Geometry: final body of the model. Coordinates: model frame, mm. Face numbers are marked on the shaded views. Give positions to 0.01 mm unless a question says otherwise; leave off trailing zeros. Write each loop counter-clockwise with the first axis right and the second up, starting at its lowest first coordinate (ties: lowest second). Pieces come first, ordered by that corner, then holes. Notation, with made-up numbers: (13, 19.25) -> (35, 19.25) arc R8 cw to (35, 25.25) -> close; hole circle Ø6 at (-12, 63.5). An arc over 180 degrees is marked (long way). Answer as a JSON object with one key per item and string values.
from build123d import *

# Parameters (mm, degrees)
PAD011_DEPTH    = 30
PAD012_DEPTH    = 0.8
PAD013_DEPTH    = 1.7
PAD014_DEPTH    = 3
CHAMFER002_SIZE = 1.5


with BuildPart() as part:
    # Sketch014 → Pad011 (new body, symmetric)
    with BuildSketch(Plane.YZ):
        with BuildLine():
            ThreePointArc((-13.5, 21.519943), (-21.311021, 27.174165), (-29.878928, 22.75))
            Line((-31.3, 22.75), (-29.878928, 22.75))
            ThreePointArc((-31.3, 24.25), (-32.05, 23.5), (-31.3, 22.75))
            Line((-31.3, 26.5), (-31.3, 24.25))
            Line((-33, 26.5), (-31.3, 26.5))
            Line((-33, 26.5), (-33, 29))
            Line((9, 29), (-33, 29))
            Line((9, 26.5), (9, 29))
            Line((9, 26.5), (6.8, 26.5))
            Line((6.8, 26.5), (6.8, 24.25))
            ThreePointArc((6.8, 22.75), (7.55, 23.5), (6.8, 24.25))
            Line((5.878928, 22.75), (6.8, 22.75))
            ThreePointArc((5.878928, 22.75), (-2.688979, 27.174165), (-10.5, 21.519943))
            Line((-13.5, 21.519943), (-10.5, 21.519943))
        make_face()
    extrude(amount=PAD011_DEPTH, both=True)

    # Sketch015 (on Face9 of Pad011) → Pad012 (join)
    with BuildSketch(Plane(origin=(0, 0, 29), x_dir=(0, -1, 0), z_dir=(0, 0, 1))):
        with BuildLine():
            ThreePointArc((-6.999999, 37.5), (-8.414213, 36.914214), (-9, 35.5))
            Line((-9, 30), (-9, 35.5))
            Line((33, 30), (-9, 30))
            Line((33, 35.5), (33, 30))
            ThreePointArc((33, 35.5), (32.414214, 36.914214), (31, 37.5))
            Line((-6.999999, 37.5), (31, 37.5))
        make_face()
        with BuildLine():
            Line((-9, -30), (33, -30))
            Line((33, -30), (33, -36))
            ThreePointArc((31, -38), (32.414214, -37.414214), (33, -36))
            Line((-7, -38), (31, -38))
            ThreePointArc((-9, -36.000001), (-8.414213, -37.414214), (-7, -38))
            Line((-9, -30), (-9, -36.000001))
        make_face()
    extrude(amount=-PAD012_DEPTH)

    # Sketch016 (on Face15 of Pad012) → Pad013 (join)
    with BuildSketch(Plane.YX.offset(-28.2)):
        with BuildLine():
            Line((-31.3, 30), (-33, 30))
            Line((-33, 30), (-33, 35.5))
            ThreePointArc((-31, 37.5), (-32.414214, 36.914214), (-33, 35.5))
            Line((6.999999, 37.5), (-31, 37.5))
            ThreePointArc((9, 35.5), (8.414213, 36.914214), (6.999999, 37.5))
            Line((9, 30), (9, 35.5))
            Line((9, 30), (6.8, 30))
            Line((6.8, 30), (6.8, 35))
            ThreePointArc((6.8, 35), (6.507107, 35.707107), (5.8, 36))
            Line((5.8, 36), (-30.3, 36))
            ThreePointArc((-30.3, 36), (-31.007107, 35.707107), (-31.3, 35))
            Line((-31.3, 30), (-31.3, 35))
        make_face()
        with BuildLine():
            ThreePointArc((7, -38), (8.414213, -37.414214), (9, -36.000001))
            Line((9, -30), (9, -36.000001))
            Line((6.8, -30), (9, -30))
            Line((6.8, -30), (6.8, -35.5))
            ThreePointArc((5.8, -36.5), (6.507107, -36.207107), (6.8, -35.5))
            Line((-30.3, -36.5), (5.8, -36.5))
            ThreePointArc((-31.3, -35.5), (-31.007107, -36.207107), (-30.3, -36.5))
            Line((-31.3, -30), (-31.3, -35.5))
            Line((-33, -30), (-31.3, -30))
            Line((-33, -36), (-33, -30))
            ThreePointArc((-33, -36), (-32.414214, -37.414214), (-31, -38))
            Line((-31, -38), (7, -38))
        make_face()
    extrude(amount=PAD013_DEPTH)

    # Sketch018 (on Face20 of Pad013) → Pad014 (join)
    with BuildSketch(Plane.YX.offset(-28.2)):
        with BuildLine():
            Line((-31.3, 35), (6.8, 35))
            ThreePointArc((6.8, 35), (6.507107, 35.707107), (5.8, 36))
            Line((5.8, 36), (-30.3, 36))
            ThreePointArc((-30.3, 36), (-31.007107, 35.707107), (-31.3, 35))
        make_face()
        with BuildLine():
            ThreePointArc((5.8, -36.5), (6.507107, -36.207107), (6.8, -35.5))
            Line((-31.3, -35.5), (6.8, -35.5))
            ThreePointArc((-31.3, -35.5), (-31.007107, -36.207107), (-30.3, -36.5))
            Line((5.8, -36.5), (-30.3, -36.5))
        make_face()
    extrude(amount=PAD014_DEPTH)

    # Chamfer002
    chamfer002_edges = [part.edges().sort_by_distance(p)[0] for p in [
        (35, -12.25, 28.2),
        (-35.5, -12.25, 28.2),
    ]]
    chamfer(chamfer002_edges, length=CHAMFER002_SIZE)


solid = part.part
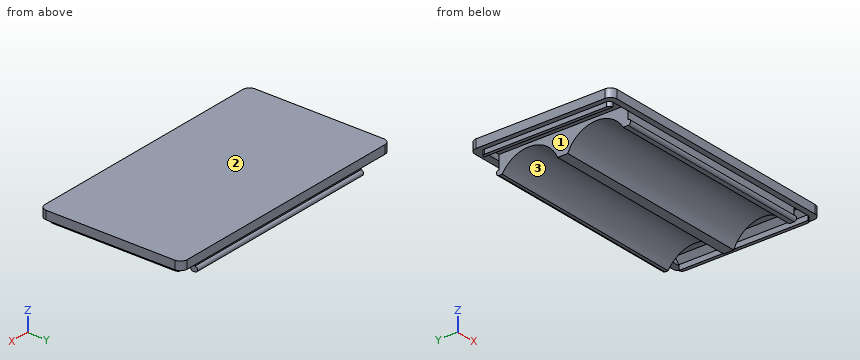
Q1. Material intervals for L1, parallel to X at y = -9, z = 25.5; L2, parallel to X at y = -23.5, z = 25.5; L3, parallel to Y at x = 13, z = 24.5, sorted ascending. Write a range as from..to.
Values:
{"L1": "-36.5..-35.5, -30..30, 35..36", "L2": "-36.5..-35.5, 35..36", "L3": "-31.3..-28.51, -15.49..-8.51, 4.51..6.8"}
Q2. First-contact query: P1, Ø4, axis at x = 19, z = 24, coming from the -Y side; P2, Ø0.7, axis at x = 5, z = 26, coming from the -Y side; P3, Ø1.8, axis at x = -13.5, z = 25, coming from the +Y side. Flat tips, straight axial feed; report the tip coordinate or a pass-through.
Values:
{"P1": "y = -32.05", "P2": "y = -31.3", "P3": "y = 7.25"}
Q3. Cut plane C-C (x = 3). Return the cut outline in (y, z).
Values:
{"outline": "(-33, 26.5) -> (-31.3, 26.5) -> (-31.3, 24.25) arc R0.75 ccw to (-31.3, 22.75) -> (-29.88, 22.75) arc R9.2 cw to (-13.5, 21.52) -> (-10.5, 21.52) arc R9.2 cw to (5.88, 22.75) -> (6.8, 22.75) arc R0.75 ccw to (6.8, 24.25) -> (6.8, 26.5) -> (9, 26.5) -> (9, 29) -> (-33, 29) -> close"}
Q4. Cut plane D-D (y = -23.5). Return the cut outline in (x, z).
Values:
{"outline": "(-38, 26.5) -> (-36.5, 26.5) -> (-36.5, 25.2) -> (-35.5, 25.2) -> (-35.5, 26.7) -> (-34, 28.2) -> (-30, 28.2) -> (-30, 27.08) -> (30, 27.08) -> (30, 28.2) -> (33.5, 28.2) -> (35, 26.7) -> (35, 25.2) -> (36, 25.2) -> (36, 26.5) -> (37.5, 26.5) -> (37.5, 29) -> (-38, 29) -> close"}
Q5. Cut plane A-A (z = 23.5). Return the cut outline in (x, y), and give its area (3 significant figures).
Values:
{"outline": "(-30, -32.05) -> (30, -32.05) -> (30, -29.37) -> (-30, -29.37) -> close; (-30, -14.63) -> (30, -14.63) -> (30, -9.37) -> (-30, -9.37) -> close; (-30, 5.37) -> (30, 5.37) -> (30, 7.55) -> (-30, 7.55) -> close", "area": "606 mm²"}
Q6. Cut plane B-B (y = -12). Return the cut outline in (x, z), and give its area (3 significant figures).
Values:
{"outline": "(-38, 26.5) -> (-36.5, 26.5) -> (-36.5, 25.2) -> (-35.5, 25.2) -> (-35.5, 26.7) -> (-34, 28.2) -> (-30, 28.2) -> (-30, 21.52) -> (30, 21.52) -> (30, 28.2) -> (33.5, 28.2) -> (35, 26.7) -> (35, 25.2) -> (36, 25.2) -> (36, 26.5) -> (37.5, 26.5) -> (37.5, 29) -> (-38, 29) -> close", "area": "475 mm²"}
Q7. Mould query, pull axis X, two halves, no side actions, for the marked faces 1, 2 and 3. Classes: pulls with the +X half, pulls with the -X half, needs draft (parallel to the pull), parting line crosses it, or undercut.
Values:
{"face 1": "undercut", "face 2": "needs draft", "face 3": "undercut"}
